from build123d import *

# Parameters (mm, degrees)
SKETCH2_R           = 29
BOSS_EXTRUDE1_DEPTH = 101
SKETCH3_R           = 2.5
BOSS_EXTRUDE2_DEPTH = 9
SKETCH4_R           = 19
BOSS_EXTRUDE3_DEPTH = 2
SKETCH5_R           = 3
BOSS_EXTRUDE4_DEPTH = 16.3


with BuildPart() as part:
    # Sketch2 → Boss-Extrude1 (new body)
    with BuildSketch(Plane(origin=(0, 0, 0), x_dir=(1, 0, 0), z_dir=(0, 1, 0))):
        with Locations(Location((0, 0, 0), (0, 0, 270))):
            Circle(SKETCH2_R)
    extrude(amount=BOSS_EXTRUDE1_DEPTH)

    # Sketch3 → Boss-Extrude2 (add)
    with BuildSketch(Plane(origin=(0, 101, 0), x_dir=(1, 0, 0), z_dir=(0, 1, 0))):
        Polygon((-29, 24), (-24, 29), (24, 29), (29, 24), (29, -24), (24, -29), (-24, -29), (-29, -24), align=None)
        with Locations(Location((-23.57, 23.57, 0), (0, 0, 270))):
            Circle(SKETCH3_R, mode=Mode.SUBTRACT)
        with Locations(Location((23.57, 23.57, 0), (0, 0, 270))):
            Circle(SKETCH3_R, mode=Mode.SUBTRACT)
        with Locations(Location((23.57, -23.57, 0), (0, 0, 270))):
            Circle(SKETCH3_R, mode=Mode.SUBTRACT)
        with Locations(Location((-23.57, -23.57, 0), (0, 0, 270))):
            Circle(SKETCH3_R, mode=Mode.SUBTRACT)
    extrude(amount=-BOSS_EXTRUDE2_DEPTH)

    # Sketch4 → Boss-Extrude3 (add)
    with BuildSketch(Plane(origin=(0, 101, 0), x_dir=(1, 0, 0), z_dir=(0, 1, 0))):
        with Locations(Location((0, 0, 0), (0, 0, 270))):
            Circle(SKETCH4_R)
    extrude(amount=BOSS_EXTRUDE3_DEPTH)

    # Sketch5 → Boss-Extrude4 (add)
    with BuildSketch(Plane(origin=(0, 103, 0), x_dir=(1, 0, 0), z_dir=(0, 1, 0))):
        with Locations(Location((0, 0, 0), (0, 0, 270))):
            Circle(SKETCH5_R)
    extrude(amount=BOSS_EXTRUDE4_DEPTH)


solid = part.part
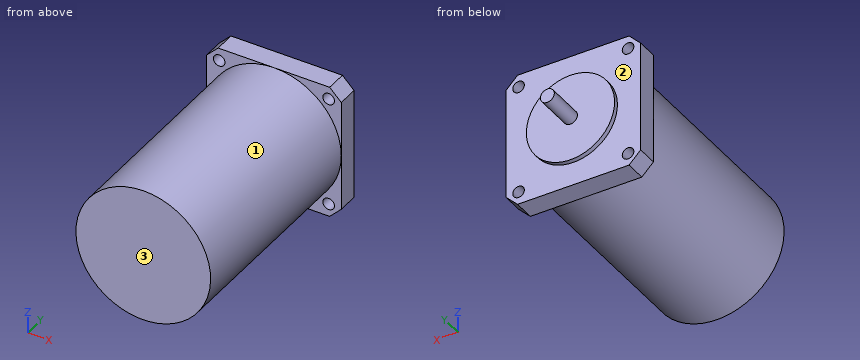
Input: part model. Units: mm. Frame: model coordinates. Face numbers are marked on the shaded views. A direction names the side the tool comes from. Round coordinates to 2 decimals unless told otherwise and drop trailing zeros. Order: outer loops, then holes, each group sorted by start corner. A loop starts at its lowest first (then second) coordinate and runs counter-clockwise, first axis right, second up. Notation, with made-up numbers: (-36, 72) - (-9, 72) arc R25 cw to (-9, 93) - close; hole circle Ø10 at (71, -17.5). An arc over 180 degrees is marked (long way). Answer as a JSON object with one key per item and string values. Group by question number.
(1) Pin query (flat end, axial travel): P1, Ø5, axis at x = -19.5, z = 21, coming from the +Y side; P2, Ø12, axis at x = -7.5, y = 40, coming from the +Z side; P3, Ø8, axis at x = 2, z = 15, coming from the +Y side. Return the tip coordinate at first contact, or that it passes through.
(2) Material intervals for probe 1 along X at (y, z) = (97, -23.57); probe 2 along Z at (x, y) = (23, 96), sorted ascending. Write a range as from..to.
(3) Cut plane C-C (y = 32.5). Return loops of the section in (x, z), then the cut area to 3 significant figures.
(4) Cut plane B-B (z = -16.5). Return loops of the section in (x, y).
(5) Reachability of the marked faces 1, 2 and 3 from +Z, -Z, +X, -X, +Y, -Y: full face, straight path, thin tool, end or side. Return the list, or none.
(6) Cut plane A-A (x = -10). Return loops of the section in (y, z), then the cut area to 3 significant figures.
Here are the results:
{
 "1": {"P1": "stops at y = 101", "P2": "stops at z = 28.96", "P3": "stops at y = 103"},
 "2": {"probe 1": "x = -29..-26.07, -21.07..21.07, 26.07..29", "probe 2": "z = -29..-26, -21.14..21.14, 26..29"},
 "3": {"outline": "circle Ø58 at (0, 0)", "area": "2,640 mm^2"},
 "4": {"outline": "(-29, 92) - (-23.85, 92) - (-23.85, 0) - (23.85, 0) - (23.85, 92) - (29, 92) - (29, 101) - (9.42, 101) - (9.42, 103) - (-9.42, 103) - (-9.42, 101) - (-29, 101) - close"},
 "5": {"face 1": "-Y", "face 2": "+Y", "face 3": "+Z, -Z, +X, -X, -Y"},
 "6": {"outline": "(0, -27.22) - (92, -27.22) - (92, -29) - (101, -29) - (101, -16.16) - (103, -16.16) - (103, 16.16) - (101, 16.16) - (101, 29) - (92, 29) - (92, 27.22) - (0, 27.22) - close", "area": "5,600 mm^2"}
}
